Geometry check sheet. Reference: drawing and pictorial views, mm from the part's lowest x, y, z. A direction names the side the tool comes from. Give positions to 0.01 mm unless a question says otherwise; leave off trailing zeros. Order: outer loops, then holes, each group sorted by start corner. A loop starts at its lowest first (then second) coordinate and runs counter-clockwise, first axis right, second up.
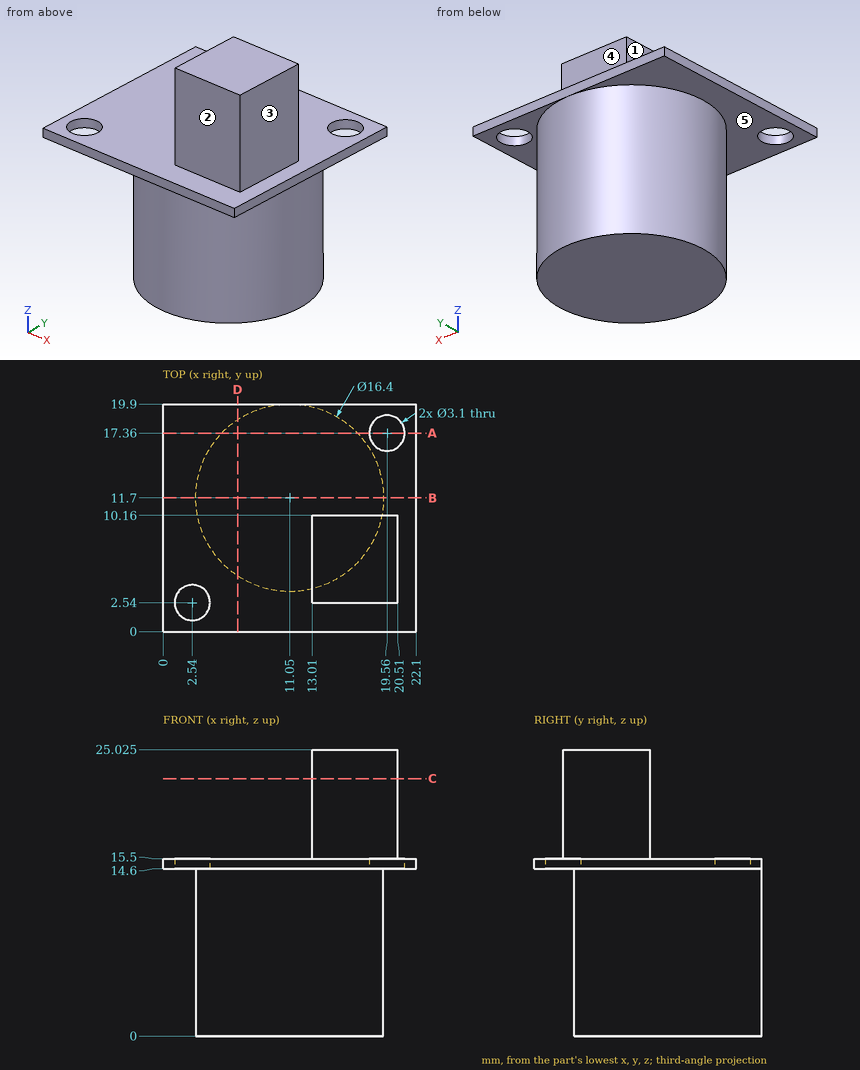
(1) Cross-section at D-D on x = 6.5. Enter the section's corners in (y, z), then the cut area to 3 significant figures.
Response values:
outline: (0, 14.6) - (4.88, 14.6) - (4.88, 0) - (18.52, 0) - (18.52, 14.6) - (19.9, 14.6) - (19.9, 15.5) - (0, 15.5) - close
area: 217 mm2
(2) Material ranges on L1, parallel to Y at x = 2.54, z = 14.95; L2, parallel to Y at x = 19.56, z = 15.1; L3, parallel to Z at x = 1.5, y = 1, recorded low to high.
Response values:
L1: y = 0 to 0.99, 4.09 to 19.9
L2: y = 0 to 15.81, 18.91 to 19.9
L3: z = 14.6 to 15.5
(3) Cross-section at A-A on y = 17.36. Enter the section's corners in (x, z).
Response values:
outline: (0, 14.6) - (5.12, 14.6) - (5.12, 0) - (16.98, 0) - (16.98, 14.6) - (18.01, 14.6) - (18.01, 15.5) - (0, 15.5) - close; (21.11, 14.6) - (22.1, 14.6) - (22.1, 15.5) - (21.11, 15.5) - close
(4) Set-up check for the marked faces 1, 2, 3, 4 and 5: record each of +Z, -Z, +X, -X, +Y, -Y from which the full face is reachable in a straight line by a thin tool's end or side.
Response values:
face 1: +Z, -X, +Y, -Y
face 2: +Z, +X, -X, -Y
face 3: +Z, +X, +Y, -Y
face 4: +Z, +X, -X, +Y
face 5: -Z
(5) Gauge pin test, flat ends, axial feed: pin 1 Ø4 at (x, z) = (18.5, 21) entering from +Y; pin 2 Ø6 at (y, z) = (6.5, 19) entering from -X; pin 3 Ø3.5 at (x, y) = (2.54, 2.54) entering from -Z. Record the tip position at first contact, or that the pin passes through.
Response values:
pin 1: stops at y = 10.16
pin 2: stops at x = 13.01
pin 3: stops at z = 14.6
(6) Cross-section at C-C on z = 22.5. Enter the section's corners in (x, y).
Response values:
outline: (13.01, 2.54) - (20.51, 2.54) - (20.51, 10.16) - (13.01, 10.16) - close
(7) Cross-section at B-B on y = 11.7. Enter the section's corners in (x, z).
Response values:
outline: (0, 14.6) - (2.85, 14.6) - (2.85, 0) - (19.25, 0) - (19.25, 14.6) - (22.1, 14.6) - (22.1, 15.5) - (0, 15.5) - close
